Here's how the part is built. I have some questions about the finished solid (model axes, mm). A direction names the side the tool comes from. Round coordinates to 2 decimals unless told otherwise and drop trailing zeros. Order: outer loops, then holes, each group sorted by start corner. A loop starts at its lowest first (then second) coordinate and runs counter-clockwise, first axis right, second up. Notation, with made-up numbers: (42.25, -6.5) -> (97.25, -6.5) arc R30 cw to (97.25, 22.5) -> close; hole circle Ø4 at (-16, -22). An arc over 180 degrees is marked (long way). Answer in a Markdown table with one row per item.
```python
from build123d import *

# Parameters (mm, degrees)
F1_DEPTH = 25
F2_W     = 7.596032
F2_H     = 21.10009
F2_W_2   = 10.268714
F2_H_2   = 30.102797
F3_DEPTH = 25
F4_R     = 2
F5_DEPTH = 35
F7_DEPTH = 3


with BuildPart() as f1:
    # F0 (on Front) → F1 (new body)
    with BuildSketch(Plane.XZ):
        Polygon((-11.404762, -2.895238), (-8.3, 0), (8.5, 0), (11.604762, -2.895238), (8.5, -6), (12.742641, -10.242641), (22.464761, -0.520521), (11.5, 10.44424), (-11.3, 10.44424), (-22.264761, -0.520521), (-12.542641, -10.242641), (-8.3, -6), align=None)
    extrude(amount=F1_DEPTH)

    # F2 (on face) → F3 (cut)
    with BuildSketch(Plane.XZ.offset(25)):
        with Locations((-20.202778, -0.557668)):
            Rectangle(F2_W, F2_H)
        with Locations((21.739119, -1.542339)):
            Rectangle(F2_W_2, F2_H_2)
    extrude(amount=-F3_DEPTH, mode=Mode.SUBTRACT)

    # F4 (on face) → F5 (cut)
    with BuildSketch(Plane.YZ.offset(16.604762)):
        with Locations((-12.5, -0.695238)):
            Circle(F4_R)
    extrude(amount=-F5_DEPTH, mode=Mode.SUBTRACT)

    # F6 (on face) → F7 (cut)
    with BuildSketch(Plane(origin=(-16.404762, 0, 0), x_dir=(0, -1, 0), z_dir=(-1, 0, 0))):
        Polygon((15.321942, -3.588329), (16.416462, 0.30209), (13.59452, 3.195181), (9.678058, 2.197854), (8.583538, -1.692565), (11.40548, -4.585657), align=None)
    extrude(amount=-F7_DEPTH, mode=Mode.SUBTRACT)


solid = f1.part
```
1. For faces 1 (the face through (-14.926, -15.025, 1.728)), 2 (the face through (-9.874, -9.547, -1.468)), 3 (the face through (14.647, -12.325, -8.339)), 4 (the face through (10.6, -12.3, -8.1)), which set-ups out of +Z, -Z, +X, -X, +Y, -Y let a thin tool reach every point of the face, with its end or its side?
Numbers:
| item | result |
|---|---|
| face 1 | -X |
| face 2 | +Y, -Y |
| face 3 | -Z, +X, +Y, -Y |
| face 4 | -Z, +Y, -Y |
2. Please list where these lines run through material, in increasing order: line 1 along Y through (x, z) = (11.5, -0.75); line 2 along Z through (x, y) = (3, -12.5); line 3 along X through (y, z) = (-17.5, -4).
Numbers:
| item | result |
|---|---|
| line 1 | y = -25 to -14.5, -10.5 to 0 |
| line 2 | z = 1.3 to 10.44 |
| line 3 | x = -16.4 to -10.3, 10.5 to 16.6 |
3. Suppose I cut it at A-A on y = -12.5. Write out the boundary of the cut face in (x, z), then the cut area to 3 significant figures.
Numbers:
| item | result |
|---|---|
| outline | (-16.4, -6.38) -> (-12.54, -10.24) -> (-8.3, -6) -> (-11.4, -2.9) -> (-11.19, -2.7) -> (-13.4, -2.7) -> (-13.4, -4.31) -> (-16.4, -4.31) -> close; (-16.4, 2.92) -> (-13.4, 2.92) -> (-13.4, 1.3) -> (16.6, 1.3) -> (16.6, 5.34) -> (11.5, 10.44) -> (-11.3, 10.44) -> (-16.4, 5.34) -> close; (8.5, -6) -> (12.74, -10.24) -> (16.6, -6.38) -> (16.6, -2.7) -> (11.39, -2.7) -> (11.6, -2.9) -> close |
| area | 345 mm2 |
4. Suppose I cut it at B-B on z = -7.5. Write out the boundary of the cut face in (x, y), then the cut area to 3 significant figures.
Numbers:
| item | result |
|---|---|
| outline | (-15.29, -25) -> (-9.8, -25) -> (-9.8, 0) -> (-15.29, 0) -> close; (10, -25) -> (15.49, -25) -> (15.49, 0) -> (10, 0) -> close |
| area | 274 mm2 |
5. We'd pull the mould along Y, two halves only. Please class faces 5 (the face through (10, -9.5, -1.4)), 6 (the face through (-14.93, -9.14, 0.28)), 7 (the face through (-14.93, -15.86, -1.67)), 8 (the face through (0, -25, 3)): released by +Y, released by -Y, zero draft, split by the parting line, or undercut.
Numbers:
| item | result |
|---|---|
| face 5 | zero draft |
| face 6 | undercut |
| face 7 | undercut |
| face 8 | released by -Y |
6. For pin 1 Ø11.5 at (x, y) = (2.5, -4) entering from -Z, with a flat end and sliding along its axis, tell me the tip position at first contact or that it passes through.
Numbers:
| item | result |
|---|---|
| pin 1 | stops at z = 0 |
7. Suppose I cut it at D-D on y = -7.5. Write out the boundary of the cut face in (x, z).
Numbers:
| item | result |
|---|---|
| outline | (-16.4, -6.38) -> (-12.54, -10.24) -> (-8.3, -6) -> (-11.4, -2.9) -> (-8.3, 0) -> (8.5, 0) -> (11.6, -2.9) -> (8.5, -6) -> (12.74, -10.24) -> (16.6, -6.38) -> (16.6, 5.34) -> (11.5, 10.44) -> (-11.3, 10.44) -> (-16.4, 5.34) -> close |
8. Suppose I cut it at C-C on x = 10.5. Write out the boundary of the cut face in (y, z).
Numbers:
| item | result |
|---|---|
| outline | (-25, -8) -> (0, -8) -> (0, -4) -> (-25, -4) -> close; (-25, -1.87) -> (-14.12, -1.87) arc R2 cw (long way) to (-10.88, -1.87) -> (0, -1.87) -> (0, 10.44) -> (-25, 10.44) -> close |
